from build123d import *

# Parameters (mm, degrees)
F1_DEPTH = 31.75


with BuildPart() as f1:
    # F0 (on Right) → F1 (new body)
    with BuildSketch(Plane.YZ):
        with BuildLine():
            add(Edge.make_bspline(
                [(-31.946953, 44.640161), (-11.409624, 43.78444), (-7.131016, 56.049787), (-7.416258, 75.731389)],
                knots=[0, 0, 0, 0, 39.603276, 39.603276, 39.603276, 39.603276], degree=3))
            Line((-31.946953, 44.640161), (-38.027544, 44.640161))
            add(Edge.make_bspline(
                [(-58.759574, 75.731389), (-58.759574, 62.895566), (-58.759574, 45.781121), (-38.027544, 44.640161)],
                knots=[0, 0, 0, 0, 37.369527, 37.369527, 37.369527, 37.369527], degree=3))
            ThreePointArc((-58.759574, 75.731389), (-62.4677, 79.439515), (-66.175826, 75.731389))
            Line((-66.175826, 75.731389), (-66.175826, 34.93752))
            ThreePointArc((-66.175826, 34.93752), (-64.315954, 30.447392), (-59.825826, 28.58752))
            Line((-59.825826, 28.58752), (-53.699948, 28.58752))
            ThreePointArc((-53.699948, 28.58752), (-49.20982, 26.727648), (-47.349948, 22.23752))
            Line((-47.349948, 22.23752), (-47.349948, -73.536955))
            Line((-47.349948, -73.536955), (-18.825883, -73.536955))
            Line((-18.825883, -73.536955), (-18.825883, 22.23752))
            ThreePointArc((-18.825883, 22.23752), (-16.966011, 26.727648), (-12.475883, 28.58752))
            Line((-12.475883, 28.58752), (-6.35, 28.58752))
            ThreePointArc((-6.35, 28.58752), (-1.859872, 30.447392), (0, 34.93752))
            Line((0, 34.93752), (0, 75.731389))
            ThreePointArc((0, 75.731389), (-3.708129, 79.439518), (-7.416258, 75.731389))
        make_face()
    extrude(amount=F1_DEPTH)


solid = f1.part
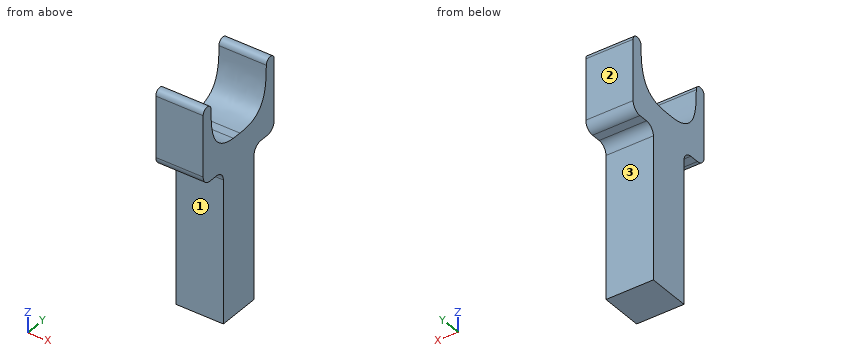
The listing builds one solid part. Answer for the finished solid, in the listing's coordinates (mm). Face numbers are marked on the shaded views. A direction names the side the tool comes from. Round coordinates to 2 decimals unless told otherwise and drop trailing zeros. Write each loop counter-clockwise with the first axis right and the second up, starting at its lowest first coordinate (ties: lowest second). Pieces come first, ordered by that corner, then holes. Notation, with made-up numbers: (18, 14.25) - (59, 14.25) arc R13 ccw to (59, 32.25) - close; hole circle Ø9 at (57.5, 2). An arc over 180 degrees is marked (long way). Use a Markdown table: item, result. Add a question column.
1. Consider line 1 (Z direction, x = 6, y = -29); line 2 (Y direction, x = 17.5, z = -25.5); line 3 (Y direction, x = 11.5, z = 55). Determine where each line is inside the solid, lowest interval first.
2. The part is cut by section A-A (z = -39). Write down the section's boundary in (x, y).
3. Flat-ended cylindrical pins translate along their axes: P1, Ø10, axis at x = 21.5, y = -41.5, coming from the +Z side; P2, Ø1.8, axis at x = 17.5, y = -35.5, coming from the +Z side; P3, Ø1.5, axis at y = -50, z = 19, coming from the -X side; P4, Ø16, axis at x = 13, z = -19.5, coming from the -Y side. Find the tip coordinate at first contact, or state that the pin passes through.
4. The part is cut by section B-B (y = -34.5). Write down the section's boundary in (x, z), and give its area (3 significant figures).
5. A tool of negligible diameter and unlimited length cuts with its end or side. For the marked faces 1, 2 and 3, from which of +Z, -Z, +X, -X, +Y, -Y can it reach the whole face along a straight path? Write none if from no direction.
Reported:
| question | item | result |
|---|---|---|
| 1 | line 1 | -73.54 to 44.61 |
| 1 | line 2 | -47.35 to -18.83 |
| 1 | line 3 | -66.18 to -55.8, -10.47 to 0 |
| 2 | outline | (0, -47.35) - (31.75, -47.35) - (31.75, -18.83) - (0, -18.83) - close |
| 3 | P1 | z = 46.34 |
| 3 | P2 | z = 44.64 |
| 3 | P3 | through |
| 3 | P4 | y = -47.35 |
| 4 | outline | (0, -73.54) - (31.75, -73.54) - (31.75, 44.64) - (0, 44.64) - close |
| 4 | area | 3,750 mm^2 |
| 5 | face 1 | -Z, +X, -X, -Y |
| 5 | face 2 | +Z, -Z, +X, -X, +Y |
| 5 | face 3 | -Z, +X, -X, +Y |
